from build123d import *

# Parameters (mm, degrees)
SKETCH1_W           = 40
SKETCH1_H           = 30
BOSS_EXTRUDE1_DEPTH = 5
SKETCH3_W           = 20
SKETCH3_H           = 30
BOSS_EXTRUDE2_DEPTH = 7.5
CUT_EXTRUDE1_DEPTH  = 39.160843806
SKETCH5_W           = 10
SKETCH5_H           = 15
CUT_EXTRUDE2_DEPTH  = 26.752603774
SKETCH6_R           = 4
CUT_EXTRUDE3_DEPTH  = 20
CHAMFER1_SIZE       = 1
FILLET1_R           = 5
SKETCH7_R           = 2
CUT_EXTRUDE4_DEPTH  = 28.386127875
CHAMFER2_SIZE       = 2
SKETCH8_R           = 32
CUT_EXTRUDE5_DEPTH  = 28.386127875


with BuildPart() as part:
    # Sketch1 → Boss-Extrude1 (new body)
    with BuildSketch(Plane(origin=(0, 0, 0), x_dir=(1, 0, 0), z_dir=(0, 1, 0))):
        Rectangle(SKETCH1_W, SKETCH1_H)
    extrude(amount=BOSS_EXTRUDE1_DEPTH)

    # Sketch3 → Boss-Extrude2 (add)
    with BuildSketch(Plane(origin=(0, 5, 0), x_dir=(1, 0, 0), z_dir=(0, 1, 0))):
        Rectangle(SKETCH3_W, SKETCH3_H)
    extrude(amount=BOSS_EXTRUDE2_DEPTH)

    # Sketch4 → Cut-Extrude1 (cut, through all)
    with BuildSketch(Plane(origin=(0, 0, -15), x_dir=(-1, 0, 0), z_dir=(0, 0, -1))):
        with BuildLine():
            Line((-10, 5), (-10, 21.180339887))
            Line((-10, 21.180339887), (10, 21.180339887))
            Line((10, 21.180339887), (10, 5))
            ThreePointArc((10, 5), (0, 11.180339887), (-10, 5))
        make_face()
    extrude(amount=-CUT_EXTRUDE1_DEPTH, mode=Mode.SUBTRACT)

    # Sketch5 → Cut-Extrude2 (cut, through all)
    with BuildSketch(Plane(origin=(0, 5, 0), x_dir=(1, 0, 0), z_dir=(0, 1, 0))):
        with Locations((-15, 7.5)):
            Rectangle(SKETCH5_W, SKETCH5_H)
        with Locations((15, 7.5)):
            Rectangle(SKETCH5_W, SKETCH5_H)
    extrude(amount=-CUT_EXTRUDE2_DEPTH, mode=Mode.SUBTRACT)

    # Sketch6 → Cut-Extrude3 (cut)
    with BuildSketch(Plane(origin=(0, 0, -15), x_dir=(-1, 0, 0), z_dir=(0, 0, -1))):
        Circle(SKETCH6_R)
    extrude(amount=-CUT_EXTRUDE3_DEPTH, mode=Mode.SUBTRACT)

    # Chamfer1
    chamfer1_edges = [part.edges().sort_by_distance(p)[0] for p in [
        (0, 11.180339887, -15),
        (-10, 2.5, -15),
        (10, 2.5, -15),
        (0, 4, -15),
    ]]
    chamfer(chamfer1_edges, length=CHAMFER1_SIZE)

    # Fillet1
    fillet1_edges = [part.edges().sort_by_distance(p)[0] for p in [
        (10, 2.5, 0),
        (-10, 2.5, 0),
    ]]
    fillet(fillet1_edges, radius=FILLET1_R)
    fillet1_2_edges = [part.edges().sort_by_distance(p)[0] for p in [
        (20, 2.5, 0),
        (-20, 2.5, 0),
    ]]
    fillet(fillet1_2_edges, radius=FILLET1_R - 0.0001)  # a hair under: the kernel refuses the full size

    # Sketch7 → Cut-Extrude4 (cut, through all)
    with BuildSketch(Plane.XZ):
        with Locations(Location((-15, 5, 0), (0, 0, 270))):
            Circle(SKETCH7_R)
        with Locations(Location((15, 5, 0), (0, 0, 270))):
            Circle(SKETCH7_R)
    extrude(amount=-CUT_EXTRUDE4_DEPTH, mode=Mode.SUBTRACT)

    # Chamfer2
    chamfer2_edges = [part.edges().sort_by_distance(p)[0] for p in [
        (20, 2.5, 15),
        (-20, 2.5, 15),
    ]]
    chamfer(chamfer2_edges, length=CHAMFER2_SIZE)

    # Sketch8 → Cut-Extrude5 (cut, through all)
    with BuildSketch(Plane.XZ):
        with Locations((0, 43)):
            Circle(SKETCH8_R)
    extrude(amount=-CUT_EXTRUDE5_DEPTH, mode=Mode.SUBTRACT)


solid = part.part
The model under review builds one solid part; all positions refer to its coordinate system, in mm. A direction names the side the tool comes from. Round coordinates to 2 decimals unless told otherwise and drop trailing zeros. Loops run counter-clockwise (first coordinate to the right, second up) from the corner with the lowest first, then second, coordinate; pieces in that order, holes last. Notation, with made-up numbers: M -15.5,-4.75 L 13.5,-4.75 A10 cw 13.5,14.25 Z; hole C 67,67 d4. An arc over 180 degrees is marked long. Answer as a JSON object with one key per item and string values.
Item 1: We need section D-D, the plane z = -7. State the section outline as (x, y) points, and give its area (3 significant figures).
Check sheet entries:
{"outline": "M -10,0 L -4,0 A4 cw 4,0 L 10,0 L 10,5 A11.18 ccw -10,5 Z", "area": "163 mm2"}
Item 2: Clearance check with flat-ended pins moving along their axes: P1, Ø5, axis at x = -14.5, z = 4, coming from the +Y side; P2, Ø4, axis at y = 7.5, z = 8.5, coming from the +X side; P3, Ø2.5, axis at x = 15, z = 5, coming from the -Y side; P4, Ø4, axis at y = 2.5, z = -9, coming from the -X side. State where each tip first meets the part, or that it passes through.
Check sheet entries:
{"P1": "y = 5", "P2": "x = 9.73", "P3": "through", "P4": "x = -10"}
Item 3: We need section C-C, the plane y = 0.75. State how many separate pieces and enclosed holes the cut face has, and give its area (3 significant figures).
Check sheet entries:
{"separate pieces": "1", "enclosed holes": "2", "area": "628 mm2"}
Item 4: We need section A-A, the plane x = 0. State the section outline as (y, z) points.
Check sheet entries:
{"outline": "M 0,5 L 4,5 L 4,-14 L 5,-15 L 10.18,-15 L 11.18,-14 L 11.18,11 L 0,11 Z"}
Item 5: The part is to be moulded in two halves that separate along X. For faces 1 (the face through (-20, 2, 9)), 2 (the face through (14, 5, 7)), 3 (the face through (0, 4, 11)), 4 (the face through (-0.16, 10.35, -14.83)), say which applies: +X half, -X half, draft (parallel to the pull), parting line (faces both ways), or undercut.
Check sheet entries:
{"face 1": "-X half", "face 2": "draft", "face 3": "undercut", "face 4": "parting line"}
Item 6: Tool access review of faces 5 (the face through (-19, 2, 14)), 6 (the face through (-14, 5, 7)), 7 (the face through (0, 2, 5)): name each direction out of +Z, -Z, +X, -X, +Y, -Y from which nothing blocks a thin tool from reaching the whole face with its end or side.
Check sheet entries:
{"face 5": "+Z, -X, +Y, -Y", "face 6": "+Z, -Z, -X, +Y", "face 7": "-Z, -Y"}
Item 7: For line 1 along Y through (x, z) = (-18, 9.5); line 2 along Y through (x, z) = (-5, 7.5); line 3 along X through (y, z) = (1.75, -10), list the stretches that pass through material, from the lowest coordinate up.
Check sheet entries:
{"line 1": "0 to 5", "line 2": "0 to 10", "line 3": "-10 to -3.6, 3.6 to 10"}
Item 8: We need section B-B, the plane z = 9. State the section outline as (x, y) points.
Check sheet entries:
{"outline": "M -20,0 L 20,0 L 20,5 L 10,5 A11.18 ccw -10,5 L -20,5 Z"}
